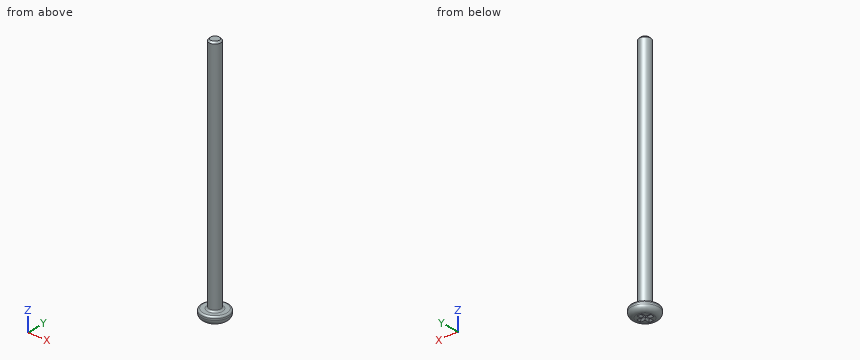
Autodesk Inventor part; units mm, degrees
ref_plane "YZ Plane" through (0, 0, 0) normal (1, 0, 0) x (0, 1, 0)
ref_plane "XZ Plane" through (0, 0, 0) normal (0, 1, 0) x (-1, 0, 0)
ref_plane "XY Plane" through (0, 0, 0) normal (0, 0, 1) x (1, 0, 0)
sketch "Sketch1" plane through (0, 0, 0) normal (0, 0, 1) x (1, 0, 0)
  circle A0 centre (0, 0) radius 4
  dimension "d0" = 8
extrude "Extrusion1" add sketch "Sketch1" along normal blind 2.5
sketch "Sketch2" plane through (0, 0, 2.5) normal (0, 0, 1) x (1, 0, 0)
  circle A0 centre (0, 0) radius 1.75
  dimension "d3" = 3.5
extrude "Extrusion2" add sketch "Sketch2" along normal blind 70
thread "Thread1"
chamfer "Chamfer1" distance 0.5 angle 45 1 edges at (-1.75, 0, 72.5)
fillet "Fillet1" radius 0.5 1 edges at (-1.75, 0, 2.5)
fillet "Fillet2" radius 1.5 1 edges at (-4, 0, 0)
sketch "Sketch3" plane through (0, 0, 0) normal (0, 0, -1) x (-1, 0, 0)
  line L0 (-1.9955, 1.419) -> (0.9534, 1.419) construction
  line L1 (0.9534, 1.419) -> (0.9534, -1.1751) construction
  line L2 (0.9534, -1.1751) -> (-1.9955, -1.1751) construction
  line L3 (-1.9955, -1.1751) -> (-1.9955, 1.419) construction
  line L4 (1.5864, -0.3671) -> (0.2314, -0.3671)
  line L5 (0.2314, -0.3671) -> (0.2314, -1.722)
  line L6 (0.2314, -1.722) -> (-0.2159, -1.722)
  line L7 (-0.2159, -1.722) -> (-0.2159, -0.3671)
  line L8 (-0.2159, -0.3671) -> (-1.5708, -0.3671)
  line L9 (-1.5708, -0.3671) -> (-1.5708, 0.064)
  line L10 (-1.5708, 0.064) -> (-0.2159, 0.064)
  line L11 (-0.2159, 0.064) -> (-0.2159, 1.419)
  line L12 (-0.2159, 1.419) -> (0.2314, 1.419)
  line L13 (0.2314, 1.419) -> (0.2314, 0.064)
  line L14 (0.2314, 0.064) -> (1.5864, 0.064)
  line L15 (1.5864, 0.064) -> (1.5864, -0.3671)
  point P0 (0, 0)
emboss "Emboss1" sketch "Sketch3" operation cut depth 2 direction (0, 0, 1)
chamfer "Chamfer2" distance 0.5 angle 45 12 edges at (-1.5864, -0.1515, 0) (-0.9089, -0.3671, 0) (-0.2314, -1.0445, 0) (-0.0078, -1.722, 0) (0.2159, -1.0445, 0) (0.8934, -0.3671, 0) (1.5708, -0.1515, 0) (0.8934, 0.064, 0) (0.2159, 0.7415, 0) (-0.0078, 1.419, 0) (-0.2314, 0.7415, 0) (-0.9089, 0.064, 0)
fillet "Fillet3" radius 0.5 1 edges at (-4, 0, 2.5)
properties part number "screw" material "Aluminum"
Geometry check sheet. Reference: the model listing, model coordinates, mm. Give positions to 0.01 mm unless a question says otherwise; leave off trailing zeros. Loops run counter-clockwise (first coordinate to the right, second up) from the corner with the lowest first, then second, coordinate; pieces in that order, holes last.
(1) Depth check by flat-ended pin: pin 1 Ø1.6 at (x, y) = (0.5, -1) entering from -Z; pin 2 Ø1 at (x, z) = (0, 44.5) entering from -Y; pin 3 Ø1.1 at (y, z) = (1, 1.5) entering from -X; pin 4 Ø0.7 at (x, z) = (1, 1.5) entering from +Y. Enter the tip coordinate at first touch or a pass-through.
From the geometry:
pin 1: stops at z = 0
pin 2: stops at y = -1.75
pin 3: stops at x = -3.97
pin 4: stops at y = 3.95
(2) Section check A-A on z = 51. Record the cut outline in (x, y), then the cut area to 3 significant figures.
From the geometry:
outline: circle Ø3.5 at (0, 0)
area: 9.62 mm2
(3) Thickness scan on L1, parallel to Z at x = 2.25, y = 1.5; L2, parallel to Z at x = -2, y = -3; L3, parallel to Y at x = 0.75, z = 35.5. Record the ranges inside material, lowest first.
From the geometry:
L1: z = 0.01 to 2.5
L2: z = 0.49 to 2.49
L3: y = -1.58 to 1.58
